Geometry check sheet. Reference: the model listing, model coordinates, mm. Coordinates: 2 decimals unless noted, no trailing zeros. Loops run counter-clockwise (first coordinate to the right, second up) from the corner with the lowest first, then second, coordinate; pieces in that order, holes last.
Autodesk Inventor part; units mm, degrees
ref_plane "YZ Plane" through (0, 0, 0) normal (1, 0, 0) x (0, 1, 0)
ref_plane "XZ Plane" through (0, 0, 0) normal (0, 1, 0) x (-1, 0, 0)
ref_plane "XY Plane" through (0, 0, 0) normal (0, 0, 1) x (1, 0, 0)
sketch "Sketch1" plane through (0, 0, 0) normal (1, 0, 0) x (0, 1, 0)
  circle A0 centre (0, 0) radius 62.5 construction
  circle A1 centre (-143.0555, 7.5) radius 50 construction
  line L0 (-143.0555, 7.5) -> (0, 0) construction
  line L1 (-161.7434, -42.5) -> (-102.4467, -42.5) construction
  line L2 (-16.0459, -62.5) -> (40.9165, -62.5) construction
  line L3 (-160.8345, -6.0612) -> (-142.874, -14.8599)
  line L4 (-142.874, -14.8599) -> (-73.1769, -16.662)
  line L5 (46.5314, -19.7571) -> (81.8069, 37.8501)
  line L6 (81.8069, 37.8501) -> (13.4998, 79.6777)
  line L7 (13.4998, 79.6777) -> (-137.4135, 83.5796)
  line L8 (-137.4135, 83.5796) -> (-176.516, 57.3036)
  line L9 (-176.516, 57.3036) -> (-160.8345, -6.0612)
  circle A2 centre (0, 0) radius 12.3
  circle A3 centre (-143.0555, 7.5) radius 12.3
  line L10 (-151.8542, -10.4606) -> (-143.0555, 7.5) construction
  arc A4 (-61.867, -16.9544) -> (-73.1769, -16.662) centre (-67.341, -9.8105) ccw construction
  line L11 (-98.4698, -16.008) -> (-97.8311, -16.0245) construction
  line L12 (-97.8311, -16.0245) -> (-61.867, -16.9544) construction
  line L13 (-61.867, -16.9544) -> (-98.4698, -16.008) construction
  line L14 (-73.1769, -16.662) -> (46.5314, -19.7571)
  line L15 (0, 0) -> (-212.6616, 0) construction
  circle A5 centre (-83.0555, 6.6011) radius 4.25
  dimension "d0" = 125
  dimension "d1" = 100
  dimension "d2" = 143.252
  dimension "d3" = 20
  dimension "d4" = 20
  dimension "d5" = 24.6
  dimension "d6" = 24.6
  dimension "d7" = 23.099
  dimension "d8" = 20
  dimension "d9" = 130
  dimension "d10" = 110
  dimension "d12" = 155.381
  dimension "d13" = 80
  dimension "d14" = 90
  dimension "d15" = 150
  dimension "Height" = 75
  dimension "d17" = 50
  dimension "d18" = 60
  dimension "d30" = 8.5
  dimension "d31" = 23
  dimension "d32" = 60
extrude "Extrusion1" add sketch "Sketch1" along normal blind 4
fillet "Fillet3" radius 10 6 edges at (2, 81.8069, 37.8501) (2, 46.5314, -19.7571) (2, -142.874, -14.8599) (2, -160.8345, -6.0612) (2, -176.516, 57.3036) (2, -137.4135, 83.5796)
chamfer "Chamfer1" distance 32 angle 45 1 edges at (2, 13.4998, 79.6777)
fillet "Fillet4" radius 10 2 edges at (2, 40.7898, 62.9668) (2, -18.4895, 80.5048)
sketch "Sketch2" plane through (4, 0, 0) normal (1, 0, 0) x (0, 0, -1)
  circle A0 centre (0, 0) radius 16.3
  circle A1 centre (0, 0) radius 12.3
  circle A2 centre (-71.4855, -128.5174) radius 4.25
  line L0 (-81.8006, -140.0609) -> (-61.209, -170.7042)
  line L1 (-50.5066, -174.8339) -> (1.5347, -161.9548)
  circle A3 centre (-35.2054, 70.8067) radius 4.25
  arc A4 (-29.322, 76.5847) -> (-43.0723, 73.2788) centre (-34.5442, 68.0566) ccw
  line L2 (14.8333, 49.5464) -> (-29.322, 76.5847)
  line L3 (-43.0723, 73.2788) -> (-62.2792, 41.9126)
  circle A5 centre (-58.9603, -53.5174) radius 4.25
  line L4 (-58.9603, -53.5174) -> (-71.4855, -128.5174)
  line L5 (-80.5388, -19.8056) -> (-83.4971, -134.225)
  point P0 (18.0192, 10.7846)
  point P1 (18.8908, -9.1727)
  dimension "d39" = 32.6
  dimension "d42" = 8.5
  dimension "d43" = 15
  dimension "d44" = 50
  dimension "d45" = 8.5
  dimension "d47" = 8
  dimension "d48" = 8
  dimension "d49" = 8.5
  dimension "d50" = 8
  dimension "d51" = 75
extrude "Extrusion2" cut sketch "Sketch2" against normal blind 9.5 contours A1 | A2 | A5 | A3
properties part number "Module Plate 1" material "Aluminum 6061"
(1) Sectioned sample at A-A on y = 0. Record the cut outline in (x, z).
Findings:
outline: (0, -18.55) - (4, -18.55) - (4, -12.3) - (0, -12.3) - close; (0, 12.3) - (4, 12.3) - (4, 75.03) - (0, 75.03) - close
(2) Sectioned sample at C-C on y = -36. Record the cut outline in (x, z), and give its area (3 significant figures).
Findings:
outline: (0, -17.62) - (4, -17.62) - (4, 80.96) - (0, 80.96) - close
area: 394 mm2
(3) Gauge pin test, flat ends, axial feed: pin 1 Ø1.5 at (x, z) = (3, 22.5) entering from +Y; pin 2 Ø2 at (x, z) = (1.5, 10) entering from -Y. Record the tip position at first contact, or that the pin passes through.
Findings:
pin 1: stops at y = 72.87
pin 2: stops at y = -165.06
(4) Sectioned sample at B-B on x = 1. Record the cut outline in (y, z), and give its area (3 significant figures).
Findings:
outline: (-174.83, 50.51) - (-161.95, -1.53) arc R10 ccw to (-156.65, -8.11) - (-144.83, -13.9) arc R10 ccw to (-140.69, -14.92) - (-73.18, -16.66) - (40.76, -19.61) arc R10 ccw to (49.55, -14.83) - (76.58, 29.32) arc R10 ccw to (73.28, 43.07) - (41.91, 62.28) arc R10 ccw to (39.53, 63.34) - (-17.23, 80.13) arc R10 ccw to (-19.81, 80.54) - (-134.22, 83.5) arc R10 ccw to (-140.06, 81.8) - (-170.7, 61.21) arc R10 ccw to start; hole circle Ø24.6 at (-143.06, 7.5); hole circle Ø8.5 at (-128.52, 71.49); hole circle Ø8.5 at (-83.06, 6.6); hole circle Ø8.5 at (-53.52, 58.96); hole circle Ø24.6 at (0, 0); hole circle Ø8.5 at (70.81, 35.21)
area: 20,400 mm2
(5) Draft check along Z on faces 1 (the cylindrical face through (2.028, -50.645, 62.093)), 2 (the flat face through (0, -50, 33)), 3 (the flat face through (1.97, -155.17, 71.65)), 4 (the flat face through (1.972, -150.823, -10.966)). Enter one of: +Z half, -Z half, draft (parallel to the pull), parting line (faces both ways), or undercut.
Findings:
face 1: undercut
face 2: draft
face 3: +Z half
face 4: -Z half
(6) Scan lines: L1, parallel to Z at x = 0.6, y = -132; L2, parallel to Y at x = 1.8, z = 8.5; L3, parallel to Y at x = 1.85, z = 61.5. Record each from-to range of solid material in increasing order.
Findings:
L1: z = -15.14 to 2.11, 12.89 to 69.05, 73.92 to 83.44
L2: y = -164.44 to -155.31, -130.8 to -86.86, -79.25 to -8.89, 8.89 to 63.83
L3: y = -170.27 to -56.93, -50.11 to 43.19
